from build123d import *

# Parameters (mm, degrees)
F1_DEPTH = 30
F2_T     = -2
F4_W     = 31
F4_H     = 26
F5_DEPTH = 4


with BuildPart() as f1:
    # F0 (on Front) → F1 (new body)
    with BuildSketch(Plane.XZ):
        with BuildLine():
            ThreePointArc((5, 0), (1.4644660941, 1.4644660941), (0, 5))
            Line((0, 5), (0, 47))
            Line((0, 47), (-35, 47))
            Line((-35, 47), (-35, 0))
            Line((-35, 0), (-10, 0))
            Line((-10, 0), (-10, -5))
            ThreePointArc((-10, -5), (-8.5355339059, -8.5355339059), (-5, -10))
            Line((-5, -10), (65, -10))
            ThreePointArc((65, -10), (68.5355339059, -8.5355339059), (70, -5))
            Line((70, -5), (70, 65))
            ThreePointArc((70, 65), (68.5355339059, 68.5355339059), (65, 70))
            Line((65, 70), (60, 70))
            Line((60, 70), (60, 95))
            Line((60, 95), (13, 95))
            Line((13, 95), (13, 60))
            Line((13, 60), (55, 60))
            ThreePointArc((55, 60), (58.5355339059, 58.5355339059), (60, 55))
            Line((60, 55), (60, 5))
            ThreePointArc((60, 5), (58.5355339059, 1.4644660941), (55, 0))
            Line((55, 0), (5, 0))
        make_face()
    extrude(amount=F1_DEPTH)

    # F2
    f2_openings = [f1.faces().sort_by_distance(p)[0] for p in [
        (13, -15, 77.5),
    ]]
    offset(amount=F2_T, openings=f2_openings, kind=Kind.INTERSECTION)

    # F4 (on offset) → F5 (cut)
    with BuildSketch(Plane.XY.offset(47)):
        with Locations((-17.5, -15)):
            Rectangle(F4_W, F4_H)
    extrude(amount=-F5_DEPTH, mode=Mode.SUBTRACT)


solid = f1.part
Source: CAD feature listing. Evaluate the final solid. Frame: model axes, mm. A direction names the side the tool comes from. Give positions to 0.01 mm unless a question says otherwise; leave off trailing zeros. Order: outer loops, then holes, each group sorted by start corner. A loop starts at its lowest first (then second) coordinate and runs counter-clockwise, first axis right, second up. Notation, with made-up numbers: (88.5, 40) -> (106.5, 40) arc R24 cw to (106.5, 50) -> close; hole circle Ø5 at (-23.5, 76). An arc over 180 degrees is marked (long way). Use a Markdown table: item, result.
1) Section query D-D, the plane x = -28. Return the cut outline in (y, z), then the cut area to 3 significant figures.
Answer list:
| item | result |
|---|---|
| outline | (-30, 0) -> (0, 0) -> (0, 47) -> (-2, 47) -> (-2, 2) -> (-28, 2) -> (-28, 47) -> (-30, 47) -> close |
| area | 240 mm² |
2) Section query A-A, the plane x = 37. Return the cut outline in (y, z).
Answer list:
| item | result |
|---|---|
| outline | (-30, -10) -> (0, -10) -> (0, 0) -> (-30, 0) -> close; (-30, 60) -> (0, 60) -> (0, 95) -> (-30, 95) -> close; hole (-28, -8) -> (-2, -8) -> (-2, -2) -> (-28, -2) -> close; hole (-28, 62) -> (-2, 62) -> (-2, 93) -> (-28, 93) -> close |
3) Mould query, pull axis Y, two halves, no side actions, for faces 1 (the flat face through (34, -15, 60)), 2 (the flat face through (58, -15, 80)), 3 (the flat face through (-7, 0, 43)). Classes: +Y half, -Y half, draft (parallel to the pull), parting line (faces both ways), or undercut.
Answer list:
| item | result |
|---|---|
| face 1 | draft |
| face 2 | undercut |
| face 3 | +Y half |
4) Section query C-C, the plane z = 49. Return the cut outline in (x, y).
Answer list:
| item | result |
|---|---|
| outline | (60, -30) -> (70, -30) -> (70, 0) -> (60, 0) -> close; hole (62, -28) -> (68, -28) -> (68, -2) -> (62, -2) -> close |
5) Reachability of faces 4 (the flat face through (36, -15, 93)), 5 (the flat face through (13, -28.3, 81.5)), 6 (the flat face through (63, -15, 70)), 7 (the flat face through (60, -15, 30)) from +Z, -Z, +X, -X, +Y, -Y: full face, straight path, thin tool, end or side. Return the list, or none.
Answer list:
| item | result |
|---|---|
| face 4 | -X |
| face 5 | +Z, -X, +Y, -Y |
| face 6 | +Z, +X, +Y, -Y |
| face 7 | +Y, -Y |
6) Section query B-B, the plane z = 31. Return the cut outline in (x, y), then the cut area to 3 significant figures.
Answer list:
| item | result |
|---|---|
| outline | (-35, -30) -> (0, -30) -> (0, 0) -> (-35, 0) -> close; (60, -30) -> (70, -30) -> (70, 0) -> (60, 0) -> close; hole (-33, -28) -> (-2, -28) -> (-2, -2) -> (-33, -2) -> close; hole (62, -28) -> (68, -28) -> (68, -2) -> (62, -2) -> close |
| area | 388 mm² |
7) Contact query for flat-ended pins moving along their axis: P1, Ø9, axis at x = -9, y = -15.5, coming from the +Z side; P2, Ø7.5, axis at y = -15, z = 80, coming from the +X side; P3, Ø12.5, axis at y = -21.5, z = 84, coming from the -X side; P4, Ø10, axis at x = 8.5, z = 74.5, coming from the +Y side. Output: stop coordinate, or through.
Answer list:
| item | result |
|---|---|
| P1 | z = 2 |
| P2 | x = 60 |
| P3 | x = 58 |
| P4 | y = 0 |
8) Ray query, line 1 along Z through (x, y) = (37.5, -12); line 2 along X through (y, z) = (-14.5, 12); line 3 along Z through (x, y) = (7.5, -26.5). Return the intervals inside material, ascending. Write a range as [from, to].
Answer list:
| item | result |
|---|---|
| line 1 | [-10, -8], [-2, 0], [60, 62], [93, 95] |
| line 2 | [-35, -33], [-2, 0], [60, 62], [68, 70] |
| line 3 | [-10, -8], [-2, 0] |
